Model file for the job. Use its own axes, mm. A direction names the side the tool comes from. Give positions to 0.01 mm unless a question says otherwise; leave off trailing zeros. Loops run counter-clockwise (first coordinate to the right, second up) from the corner with the lowest first, then second, coordinate; pieces in that order, holes last. Notation, with made-up numbers: M -5,42 L 39,42 A27 cw 39,69 Z; hole C -39,-16.5 d5. An arc over 180 degrees is marked long. Use CSV: the item, a comma, the result in double quotes. Start each with the question number.
(1) Slice it at A-A on y = 0. List the corners of the cut face in (x, z).
(2) Slice it at D-D on x = -11.5. List the corners of the cut face in (y, z).
(3) Slice it at B-B on z = -20.5. List the corners of the cut face in (x, y), and give its area (3 significant figures).
(4) Tool access for faces 4 (the face through (-5.4, 22, -9.8)), 5 (the face through (8, -25, -13)), 6 (the face through (15, 0, 17)): list every direction of +Z, -Z, +X, -X, +Y, -Y with a clear straight run to the whole face (end or side of a thin tool).
(5) Wall check: line 1 along X through (y, z) = (-16, -10); line 2 along X through (y, z) = (0, 3); line 3 along Y through (x, z) = (9, -22). Give the ranges that are in metal, low to high. Write a range as from..to.
(6) Flat gauge pins, fed straight in: P1, Ø4, axis at x = 2, z = -13.5, coming from the +Y side; P2, Ø12, axis at x = -17.5, y = 4, coming from the -Z side; P3, Ø6.5, axis at x = -16, y = 0.5, coming from the -Z side; P4, Ø2.5, axis at x = -6.5, z = -20.5, coming from the -Y side. Where does each tip first touch, or does it go through?
(7) Slice it at C-C on x = 0. List the corners of the cut face in (y, z).
(8) Two-plate mould, pull along Y, no slides. Class faces 1 (the face through (0.21, 20.938, 8.956)), 2 (the face through (-8, 0, 3)), 3 (the face through (0, 19, -24)): pulls with the +Y half, pulls with the -Y half, needs draft (parallel to the pull), parting line crosses it, or undercut.
```python
from build123d import *

# Parameters (mm, degrees)
F0_W      = 60
F0_H      = 48
F0_W_2    = 8
F0_H_2    = 11
F1_DEPTH  = 23
F2_W      = 18
F2_H      = 5
F3_DEPTH  = 46.001
F5_DEPTH  = 15
F6_R      = 8
F7_DEPTH  = 48.001
F8_W      = 16
F8_H      = 28
F9_DEPTH  = 8
F10_R     = 5
F11_DEPTH = 52.001


# Not quite as in the source:
# - a pattern or mirror of a feature is missing from the dataset's text; its kind, count and spacing are read off the source's solid


with BuildPart() as f1:
    # F0 (on Right) → F1 (new body, symmetric)
    with BuildSketch(Plane.YZ):
        Rectangle(F0_W, F0_H)
        with Locations((0, 11.5)):
            Rectangle(F0_W_2, F0_H_2, mode=Mode.SUBTRACT)
    extrude(amount=F1_DEPTH, both=True)

    # F2 (on face) → F3 (cut, through all)
    with BuildSketch(Plane.YZ.offset(23)):
        with Locations((0, -21.5)):
            Rectangle(F2_W, F2_H)
    extrude(amount=-F3_DEPTH, mode=Mode.SUBTRACT)

    # F4 (on Right) → F5 (cut, symmetric)
    with BuildSketch(Plane.YZ):
        Polygon((-15, 24), (-30, 24), (-30, -14), align=None)
    f5 = extrude(amount=F5_DEPTH, both=True, mode=Mode.SUBTRACT)

    # F5_copies: F5 across plane
    add(f5.mirror(Plane.ZX), mode=Mode.SUBTRACT)

    # F6 (on face) → F7 (cut, through all)
    with BuildSketch(Plane.XY.offset(24)):
        Circle(F6_R)
    extrude(amount=-F7_DEPTH, mode=Mode.SUBTRACT)

    # F8 (on face) → F9 (cut)
    with BuildSketch(Plane.XZ.offset(30)):
        with Locations((0, -10)):
            Rectangle(F8_W, F8_H)
    f9 = extrude(amount=-F9_DEPTH, mode=Mode.SUBTRACT)

    # F9_copies: F9 across plane
    add(f9.mirror(Plane.ZX), mode=Mode.SUBTRACT)

    # F10 (on face) → F11 (cut, through all)
    with BuildSketch(Plane.XZ.offset(22)):
        with Locations((0, -10)):
            Circle(F10_R)
    extrude(amount=-F11_DEPTH, mode=Mode.SUBTRACT)


solid = f1.part
```
Reply:
1,outline,"M -23,-19 L -8,-19 L -8,6 L -23,6 Z; M -23,17 L -8,17 L -8,24 L -23,24 Z; M 8,-19 L 23,-19 L 23,6 L 8,6 Z; M 8,17 L 23,17 L 23,24 L 8,24 Z"
2,outline,"M -30,-24 L -9,-24 L -9,-19 L 9,-19 L 9,-24 L 30,-24 L 30,-14 L 15,24 L -15,24 L -30,-14 Z; hole M -4,6 L 4,6 L 4,17 L -4,17 Z"
3,outline,"M -23,-30 L -8,-30 L -8,-22 L 8,-22 L 8,-30 L 23,-30 L 23,-9 L -23,-9 Z; M -23,9 L 23,9 L 23,30 L 8,30 L 8,22 L -8,22 L -8,30 L -23,30 Z"
3,area,"1,680 mm^2"
4,face 4,"-Z, +Y"
4,face 5,"-Z, -Y"
4,face 6,"+X, -X"
5,line 1,"x = -23..-5, 5..23"
5,line 2,"x = -23..-8, 8..23"
5,line 3,"y = -30..-9, 9..30"
6,P1,"stops at y = 22"
6,P2,"stops at z = -24"
6,P3,"stops at z = -19"
6,P4,"stops at y = -22"
7,outline,"M -22.89,4 L -22,4 L -22,-5 L -8,-5 L -8,24 L -15,24 Z; M -22,-24 L -9,-24 L -9,-19 L -8,-19 L -8,-15 L -22,-15 Z; M 8,-19 L 9,-19 L 9,-24 L 22,-24 L 22,-15 L 8,-15 Z; M 8,-5 L 22,-5 L 22,4 L 22.89,4 L 15,24 L 8,24 Z"
8,face 1,"pulls with the +Y half"
8,face 2,"undercut"
8,face 3,"needs draft"
